CAD build for the part. Positions are in the model's coordinates, mm. Face numbers are marked on the shaded views. A direction names the side the tool comes from. Give positions to 0.01 mm unless a question says otherwise; leave off trailing zeros. Write each loop counter-clockwise with the first axis right and the second up, starting at its lowest first coordinate (ties: lowest second). Pieces come first, ordered by that corner, then holes. Notation, with made-up numbers: (2, -12) -> (50, -12) arc R19 cw to (50, 14) -> close; hole circle Ø5 at (1, -30). An arc over 180 degrees is marked (long way). Answer as a JSON object with one key per item and string values.
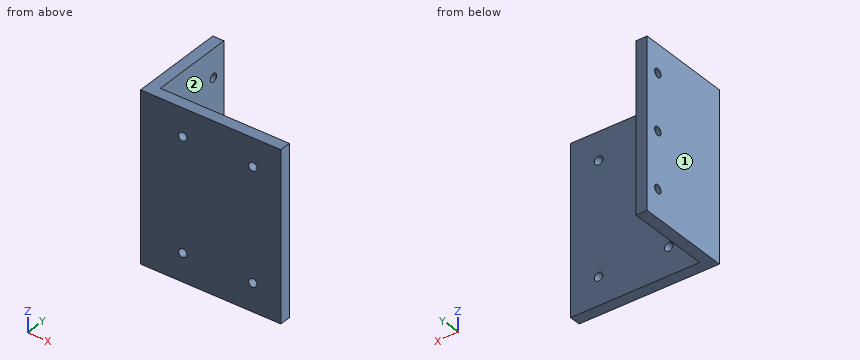
```python
from build123d import *

# Parameters (mm, degrees)
EXTRUSION1_DEPTH                = 60
ESQUISSE2_R                     = 1.5
EXTRUSION2_DEPTH                = 91.642153549
R_P_TITION_LIN_AIRE1_COUNT      = 2
R_P_TITION_LIN_AIRE1_PITCH      = 40
R_P_TITION_LIN_AIRE1_COUNT_DIR2 = 2
R_P_TITION_LIN_AIRE1_PITCH_DIR2 = 25
ESQUISSE3_W                     = 123.67499348
ESQUISSE3_H                     = 39.653502897
EXTRUSION3_DEPTH                = 10
ESQUISSE4_R                     = 1.5
EXTRUSION4_DEPTH                = 10
R_P_TITION_LIN_AIRE2_COUNT      = 3
R_P_TITION_LIN_AIRE2_PITCH      = 20


with BuildPart() as part:
    # Esquisse1 → Extrusion1 (new body)
    with BuildSketch(Plane.XY):
        Polygon((0, 0), (4, 0), (50, 0), (50, 4), (4, 4), (4, 50), (0, 50), align=None)
    extrude(amount=EXTRUSION1_DEPTH)

    # Esquisse2 → Extrusion2 (cut, through all)
    with BuildSketch(Plane(origin=(0, 4, 0), x_dir=(1, 0, 0), z_dir=(0, 1, 0))):
        with Locations(Location((40, -50, 0), (0, 0, 270))):
            Circle(ESQUISSE2_R)
    extrusion2 = extrude(amount=-EXTRUSION2_DEPTH, mode=Mode.SUBTRACT)

    # Répétition linéaire1: Extrusion2 2 × 2
    with Locations(*[(-j * R_P_TITION_LIN_AIRE1_PITCH_DIR2, 0, -i * R_P_TITION_LIN_AIRE1_PITCH) for i in range(R_P_TITION_LIN_AIRE1_COUNT) for j in range(R_P_TITION_LIN_AIRE1_COUNT_DIR2) if (i, j) != (0, 0)]):
        add(extrusion2, mode=Mode.SUBTRACT)

    # Esquisse3 → Extrusion3 (cut)
    with BuildSketch(Plane.ZY):
        with Locations((37.763783115, 53.826751449)):
            Rectangle(ESQUISSE3_W, ESQUISSE3_H)
    extrude(amount=-EXTRUSION3_DEPTH, mode=Mode.SUBTRACT)

    # Esquisse4 → Extrusion4 (cut)
    with BuildSketch(Plane.ZY):
        with Locations((50, 29)):
            Circle(ESQUISSE4_R)
    extrusion4 = extrude(amount=-EXTRUSION4_DEPTH, mode=Mode.SUBTRACT)

    # Répétition linéaire2: Extrusion4 ×3
    with Locations(*[(0, 0, -i * R_P_TITION_LIN_AIRE2_PITCH) for i in range(1, R_P_TITION_LIN_AIRE2_COUNT)]):
        add(extrusion4, mode=Mode.SUBTRACT)


solid = part.part
```
1) Pin check, flat tips, straight feed: pin 1 (2.5 mm diameter, centred on x = 40, z = 50, fed in from -Y); pin 2 (4 mm diameter, centred on y = 29, z = 10, fed in from +X); pin 3 (8 mm diameter, centred on x = 30.5, z = 42, fed in from +Y). Stop position of each tip, or through.
Model answer:
{"pin 1": "passes through", "pin 2": "stops at x = 4", "pin 3": "stops at y = 4"}
2) Slice it at C-C (z = 30). List the corners of the cut face in (x, y), then the cut area to 3 significant figures.
Model answer:
{"outline": "(0, 0) -> (50, 0) -> (50, 4) -> (4, 4) -> (4, 27.5) -> (0, 27.5) -> close; (0, 30.5) -> (4, 30.5) -> (4, 34) -> (0, 34) -> close", "area": "308 mm2"}
3) Wall check: probe 1 along X at (y, z) = (2, 50); probe 2 along Y at (x, z) = (42.5, 31.5). Give the ranges that are in metal, low to high.
Model answer:
{"probe 1": "x = 0 to 13.5, 16.5 to 38.5, 41.5 to 50", "probe 2": "y = 0 to 4"}
4) Slice it at D-D (x = 15). List the corners of the cut face in (y, z), then the cut area to 3 significant figures.
Model answer:
{"outline": "(0, 0) -> (4, 0) -> (4, 8.5) -> (0, 8.5) -> close; (0, 11.5) -> (4, 11.5) -> (4, 48.5) -> (0, 48.5) -> close; (0, 51.5) -> (4, 51.5) -> (4, 60) -> (0, 60) -> close", "area": "216 mm2"}
5) Slice it at A-A (y = 29). List the corners of the cut face in (x, z).
Model answer:
{"outline": "(0, 0) -> (4, 0) -> (4, 8.5) -> (0, 8.5) -> close; (0, 11.5) -> (4, 11.5) -> (4, 28.5) -> (0, 28.5) -> close; (0, 31.5) -> (4, 31.5) -> (4, 48.5) -> (0, 48.5) -> close; (0, 51.5) -> (4, 51.5) -> (4, 60) -> (0, 60) -> close"}
6) Slice it at B-B (z = 50). List the corners of the cut face in (x, y).
Model answer:
{"outline": "(0, 0) -> (13.5, 0) -> (13.5, 4) -> (4, 4) -> (4, 27.5) -> (0, 27.5) -> close; (0, 30.5) -> (4, 30.5) -> (4, 34) -> (0, 34) -> close; (16.5, 0) -> (38.5, 0) -> (38.5, 4) -> (16.5, 4) -> close; (41.5, 0) -> (50, 0) -> (50, 4) -> (41.5, 4) -> close"}
7) 3-axis set-ups, long thin cutter, end or side, ignore diameter. For the marked faces 1 and 2: which of +Z, -Z, +X, -X, +Y, -Y reach the whole face in a straight line?
Model answer:
{"face 1": "+Z, -Z, -X, +Y, -Y", "face 2": "+Z, -Z, +X, +Y"}
